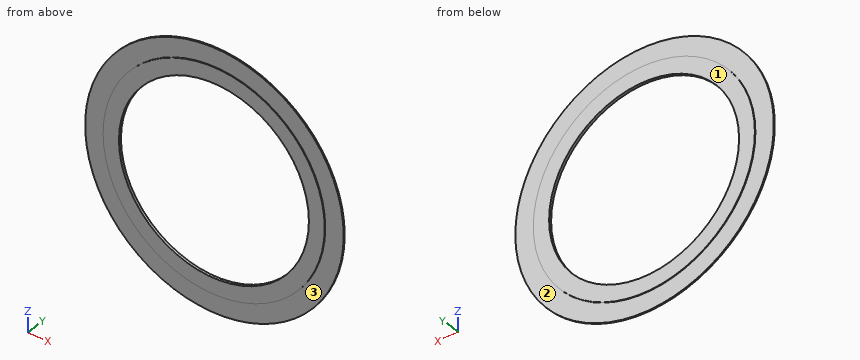
from build123d import *

# Parameters (mm, degrees)
F0_R     = 155.575
F0_R_2   = 114.3
F1_DEPTH = 1.5875
F4_R     = 133.35
F4_R_2   = 114.3
F5_DEPTH = 1.5875
F6_R     = 133.35
F6_R_2   = 114.3
F7_DEPTH = 0.79375


with BuildPart() as f1:
    # F0 (on Front) → F1 (new body)
    with BuildSketch(Plane.XZ):
        Circle(F0_R)
        Circle(F0_R_2, mode=Mode.SUBTRACT)
    extrude(amount=F1_DEPTH)

    # F4 (on offset) → F5 (join)
    with BuildSketch(Plane.XZ.offset(0.79375)):
        Circle(F4_R)
        Circle(F4_R_2, mode=Mode.SUBTRACT)
    extrude(amount=-F5_DEPTH)

    # F6 (on offset) → F7 (join)
    with BuildSketch(Plane.XZ.offset(1.5875)):
        Circle(F6_R)
        Circle(F6_R_2, mode=Mode.SUBTRACT)
    extrude(amount=F7_DEPTH)


solid = f1.part
Model file for the job. Use its own axes, mm. Face numbers are marked on the shaded views. A direction names the side the tool comes from. Round coordinates to 2 decimals unless told otherwise and drop trailing zeros. Loops run counter-clockwise (first coordinate to the right, second up) from the corner with the lowest first, then second, coordinate; pieces in that order, holes last.
1. Tool access for the marked faces 1, 2 and 3: list every direction of +Z, -Z, +X, -X, +Y, -Y with a clear straight run to the whole face (end or side of a thin tool).
Check values:
face 1: +Z, -Z, +X, -X, +Y
face 2: +Y
face 3: -Y
2. Drop flat-ended pins along their axis: P1, Ø1, axis at y = -1.5, z = 25, coming from the +X side; P2, Ø3, axis at x = -103, z = 88.5, coming from the -Y side. Give the stop position or say it passes through.
Check values:
P1: stops at x = 153.63
P2: stops at y = -1.59
3. Band-saw the part on C-C, the plane y = -1.05. List the corners of the cut face in (x, z) (3 decimals), and give its area (3 significant figures).
Check values:
outline: circle Ø311.15 at (0, 0); hole circle Ø228.6 at (0, 0)
area: 35,000 mm2
4. Band-saw the part on D-D, the plane x = 125.5. List the corners of the cut face in (y, z).
Check values:
outline: (-2.38, -45.08) - (-1.59, -45.08) - (-1.59, -91.94) - (0, -91.94) - (0, -45.08) - (0.79, -45.08) - (0.79, 45.08) - (0, 45.08) - (0, 91.94) - (-1.59, 91.94) - (-1.59, 45.08) - (-2.38, 45.08) - close
5. Wall check: probe 1 along X at (y, z) = (-2.2, -0.5); probe 2 along Z at (x, y) = (0, -0.4) (3 decimals); probe 3 along Y at (x, z) = (91.5, -123). Give the ranges that are in metal, low to high.
Check values:
probe 1: x = -133.35 to -114.3, 114.3 to 133.35
probe 2: z = -155.575 to -114.3, 114.3 to 155.575
probe 3: y = -1.59 to 0
